Geometry: final body of the model. Coordinates: model frame, mm. Coordinates: 2 decimals unless noted, no trailing zeros. Write each loop counter-clockwise with the first axis right and the second up, starting at its lowest first coordinate (ties: lowest second). Pieces come first, ordered by that corner, then holes. Notation, with made-up numbers: (86.5, 27) - (132.5, 27) arc R30 ccw to (132.5, 54) - close; hole circle Ø8 at (-27, 10). An arc over 180 degrees is marked (long way). Answer as a JSON object with one key per item and string values. Group by question number.
Item 1: Section C-C on x = -45. Return loops of the section in (y, z), and give its area (3 significant figures).
Item 2: First-contact query: pin 1 Ø1 at (y, z) = (2, 96.5) entering from +X; pin 2 Ø1 at (y, z) = (0.5, 28) entering from -X. Flat tips, straight axial feed; report the tip coordinate or a pass-through.
Item 3: Line query: line 1 along Z through (x, y) = (-32.5, 0.6); line 2 along Z through (x, y) = (38, 0.8); line 3 along Z through (x, y) = (50.5, 1.35). Output: solid intervals per line, ascending. Write a range as from..to.
Item 4: Section D-D on y = 1.3. State how many separate pieces and enclosed holes the cut face has, and give its area (3 significant figures).
Item 5: Section B-B on z = 49.5. Return loops of the section in (x, y).
Item 6: Section A-A on x = -20. Return loops of the section in (y, z).
Autodesk Inventor part; units mm, degrees
ref_plane "YZ Plane" through (0, 0, 0) normal (1, 0, 0) x (0, 1, 0)
ref_plane "XZ Plane" through (0, 0, 0) normal (0, 1, 0) x (-1, 0, 0)
ref_plane "XY Plane" through (0, 0, 0) normal (0, 0, 1) x (1, 0, 0)
sketch "スケッチ1" plane through (0, 0, 0) normal (0, 1, 0) x (-1, 0, 0)
  circle A0 centre (0, 0) radius 130
  dimension "d0" = 260
extrude "プレート1" add sketch "スケッチ1" along normal blind 2
sketch "スケッチ4" plane through (0, 2, 0) normal (0, 1, 0) x (1, 0, 0)
  circle A0 centre (0, 0) radius 130
  line L0 (-106.1838, 75) -> (-60, 40)
  line L1 (-60, 40) -> (-60, -40)
  line L2 (-60, -40) -> (-106.1838, -75)
  point P0 (-60, 0)
  dimension "d17" = 40
  dimension "d18" = 75
  dimension "d19" = 60
extrude "押し出し2" cut sketch "スケッチ4" against normal through all contours L0 L1 L2 A0 picked at (-83.3333, 0)
sketch "スケッチ7" plane through (0, 2, 0) normal (0, 1, 0) x (1, 0, 0)
  arc A0 (-106.1838, -75) -> (-106.1838, 75) centre (0, 0) ccw
  line L0 (-48.7827, 120.5) -> (48.7827, 120.5)
  line L1 (-48.7827, -120.5) -> (48.7827, -120.5)
  line L2 (105, -76.6485) -> (105, 76.6485)
  dimension "d68" = 120.5
  dimension "d69" = 120.5
  dimension "d70" = 105
extrude "押し出し4" cut sketch "スケッチ7" against normal through all
fillet "フィレット4" radius 50 6 edges at (-48.7827, 1, 120.5) (48.7827, 1, 120.5) (105, 1, -76.6485) (105, 1, 76.6485) (-48.7827, 1, -120.5) (48.7827, 1, -120.5)
sketch "スケッチ9" plane through (0, 2, 0) normal (0, 1, 0) x (1, 0, 0)
  line L0 (101.5, -60) -> (101.5, 60) construction
  line L1 (101.5, -60) -> (221.5, -60) construction
  line L2 (105, -58.0948) -> (105, 58.0948) construction
  point P0 (0, 0)
  point P1 (101.5, 0)
  dimension "d71" = 120
  dimension "d72" = 90
  dimension "d73" = 3.5
hole "穴4" at (101.5, 2, 60) at (101.5, 2, -60) direction (0, -1, 0) diameter 3.5 depth 2 tip angle 118
sketch "スケッチ10" plane through (0, 2, 0) normal (0, 1, 0) x (1, 0, 0)
  line L0 (10, -105.5) -> (-10, -105.5) construction
  line L1 (-10, -105.5) -> (-10, 105.5) construction
  line L2 (-10, 105.5) -> (10, 105.5) construction
  line L3 (10, 105.5) -> (10, -105.5) construction
  line L4 (10, -105.5) -> (-10, 105.5) construction
  line L5 (-10, -105.5) -> (10, 105.5) construction
  point P0 (0, 0)
  dimension "d81" = 20
  dimension "d82" = 211
hole "穴5" at (-10, 2, 105.5) at (10, 2, 105.5) at (10, 2, -105.5) at (-10, 2, -105.5) direction (0, -1, 0) diameter 3.5 depth 2 tip angle 118
sketch "スケッチ11" plane through (0, 2, 0) normal (0, 1, 0) x (1, 0, 0)
  line L0 (-32.5, 116.5) -> (32.5, 116.5) construction
  line L1 (-32.5, 116.5) -> (32.5, 116.5) construction
  line L2 (37.812, 120.5) -> (-37.812, 120.5) construction
  point P0 (0, 0)
  point P1 (0, 116.5)
  dimension "d90" = 65
  dimension "d91" = 0
  dimension "d92" = 4
hole "穴6" at (32.5, 2, -116.5) at (-32.5, 2, -116.5) direction (0, -1, 0) diameter 3.5 end through all
mirror "ミラー3" about plane through (0, 0, 0) normal (0, 0, 1) of "穴6"
sketch "スケッチ12" plane through (0, 2, 0) normal (0, 1, 0) x (1, 0, 0)
  line L0 (-50, 10) -> (-50, -10) construction
  line L1 (-50, 10) -> (-30, 10) construction
  line L2 (-60, 40) -> (-60, -40) construction
  point P0 (0, 0)
  point P1 (-50, 0)
  dimension "d100" = 20
  dimension "d101" = 90
  dimension "d102" = 10
hole "穴7" at (-50, 2, 10) at (-50, 2, -10) direction (0, -1, 0) diameter 3.5 end through all
sketch "スケッチ13" plane through (0, 2, 0) normal (0, 1, 0) x (1, 0, 0)
  line L0 (-10, 40) -> (40, 40) construction
  line L1 (-10, 10) -> (40, 10)
  line L2 (40, 70) -> (-10, 70)
  arc A0 (-10, 70) -> (-10, 10) centre (-10, 40) ccw
  arc A1 (40, 10) -> (40, 70) centre (40, 40) ccw
  point P0 (0, 0)
  point P1 (15, 40)
  dimension "d110" = 40
  dimension "d111" = 60
  dimension "d112" = 50
  dimension "d113" = 15
extrude "押し出し5" cut sketch "スケッチ13" against normal through all
sketch "スケッチ14" plane through (0, 2, 0) normal (0, 1, 0) x (1, 0, 0)
  line L0 (72.6777, 95.6777) -> (55, 78) construction
  line L1 (75.5061, 92.8492) -> (57.8284, 75.1716)
  line L2 (52.1716, 80.8284) -> (69.8492, 98.5061)
  arc A0 (75.5061, 92.8492) -> (69.8492, 98.5061) centre (72.6777, 95.6777) ccw
  arc A1 (52.1716, 80.8284) -> (57.8284, 75.1716) centre (55, 78) ccw
  line L3 (-10, 70) -> (40, 70)
  point P0 (0, 0)
  point P1 (63.8388, 86.8388)
  dimension "d116" = 135
  dimension "d117" = 8
  dimension "d118" = 25
  dimension "d119" = 4
  dimension "d120" = 15
extrude "押し出し6" cut sketch "スケッチ14" against normal through all
pattern_linear "矩形状パターン1" count 6 spacing 25 along (-1, 0, 0) of "押し出し6"
mirror "ミラー4" about plane through (0, 0, 0) normal (0, 0, 1) of "押し出し5", "押し出し6", "矩形状パターン1"
sketch "スケッチ15" plane through (0, 0, 0) normal (0, -1, 0) x (1, 0, 0)
  arc A0 (73.6766, 79.5874) -> (73.6766, 77.4126) centre (74.2931, 78.5) ccw
  arc A1 (74.9095, -79.5874) -> (74.9095, -77.4126) centre (74.2931, -78.5) ccw
  point P0 (0, 0)
hole "穴8" at (74.2931, 0, -78.5) at (74.2931, 0, 78.5) direction (0, 1, 0) diameter 3.5 end through all
sketch "スケッチ16" plane through (0, 2, 0) normal (0, 1, 0) x (1, 0, 0)
  arc A0 (-61.4446, 114.5625) -> (-106.1838, 75) centre (0, 0) ccw
  arc A1 (-106.1838, -75) -> (-61.4446, -114.5625) centre (0, 0) ccw
  line L0 (-102.4695, 80) -> (-102.4695, -80)
  line L1 (-102.4695, 80) -> (57.5305, 80) construction
  line L2 (-106.1838, 75) -> (-60, 40)
  line L3 (-60, -40) -> (-106.1838, -75)
  point P0 (-102.4695, 72.1852)
  point P1 (-102.4695, -72.1852)
  dimension "d133" = 160
  dimension "d134" = 90
extrude "押し出し7" cut sketch "スケッチ16" against normal through all
sketch "スケッチ17" plane through (0, 2, 0) normal (0, 1, 0) x (1, 0, 0)
  line L0 (-92.9695, 76.5) -> (-82.9695, 76.5) construction
  line L1 (-82.9695, 76.5) -> (-82.9695, -76.5) construction
  line L2 (-82.9695, -76.5) -> (-92.9695, -76.5) construction
  line L3 (-92.9695, -76.5) -> (-92.9695, 76.5) construction
  line L4 (-92.9695, 76.5) -> (-82.9695, -76.5) construction
  line L5 (-82.9695, 76.5) -> (-92.9695, -76.5) construction
  line L6 (-102.4695, 80) -> (-102.4695, 72.1852) construction
  point P0 (0, 0)
  point P1 (-87.9695, 0)
  dimension "d137" = 10
  dimension "d138" = 153
  dimension "d139" = 9.5
hole "穴9" at (-92.9695, 2, -76.5) at (-82.9695, 2, -76.5) at (-92.9695, 2, 76.5) at (-82.9695, 2, 76.5) direction (0, -1, 0) diameter 3.5 end through all
fillet "フィレット5" radius 2 6 edges at (-102.4695, 1, -72.1852) (-102.4695, 1, 80) (-102.4695, 1, -80) (-60, 1, -40) (-60, 1, 40) (-102.4695, 1, 72.1852)
sketch "スケッチ18" plane through (0, 2, 0) normal (0, 1, 0) x (1, 0, 0)
  line L0 (105, -58.0948) -> (105, 58.0948)
  line L1 (-60, 39.0062) -> (-60, -39.0062)
  line L2 (-60, 0) -> (105, 0) construction
  circle A0 centre (-50, 10) radius 1.75 construction
  line L3 (95, -10) -> (-50, -10) construction
  line L4 (-50, -10) -> (-50, 10) construction
  line L5 (-50, 10) -> (95, 10) construction
  line L6 (95, 10) -> (95, -10) construction
  line L7 (95, -10) -> (-50, 10) construction
  line L8 (-50, -10) -> (95, 10) construction
  line L9 (52.5, -5) -> (-7.5, -5) construction
  line L10 (-7.5, -5) -> (-7.5, 5) construction
  line L11 (-7.5, 5) -> (52.5, 5) construction
  line L12 (52.5, 5) -> (52.5, -5) construction
  line L13 (52.5, -5) -> (-7.5, 5) construction
  line L14 (-7.5, -5) -> (52.5, 5) construction
  point P0 (0, 0)
  point P1 (22.5, 0)
  point P2 (22.5, 0)
  dimension "d148" = 60
  dimension "d149" = 10
hole "穴10" at (95, 2, 10) at (95, 2, -10) at (52.5, 2, 5) at (52.5, 2, -5) at (-7.5, 2, -5) at (-7.5, 2, 5) direction (0, -1, 0) diameter 3.5 end through all
sketch "スケッチ19" plane through (0, 2, 0) normal (0, 1, 0) x (1, 0, 0)
  line L0 (-60, 39.0062) -> (-60, -39.0062)
  arc A0 (-60, 39.0062) -> (-60.792, 40.6002) centre (-62, 39.0062) ccw
  line L1 (-101.6775, 71.5849) -> (-60.792, 40.6002)
  arc A1 (-102.4695, 73.1789) -> (-101.6775, 71.5849) centre (-100.4695, 73.1789) ccw
  line L2 (-102.4695, 79.3088) -> (-102.4695, 73.1789)
  arc A2 (-102.0393, 80.548) -> (-102.4695, 79.3088) centre (-100.4695, 79.3088) ccw
  arc A3 (-61.4446, 114.5625) -> (-102.0393, 80.548) centre (0, 0) ccw
  arc A4 (-37.812, 120.5) -> (-61.4446, 114.5625) centre (-37.812, 70.5) ccw
  line L3 (37.812, 120.5) -> (-37.812, 120.5)
  arc A5 (61.4446, 114.5625) -> (37.812, 120.5) centre (37.812, 70.5) ccw
  arc A6 (89.375, 94.404) -> (61.4446, 114.5625) centre (0, 0) ccw
  arc A7 (105, 58.0948) -> (89.375, 94.404) centre (55, 58.0948) ccw
  line L4 (105, -58.0948) -> (105, 58.0948)
  line L5 (-60, 0) -> (105, 0)
extrude "押し出し8" cut sketch "スケッチ19" against normal through all
fillet "フィレット6" radius 1 2 edges at (-60, 1, 0) (105, 1, 0)
sketch "スケッチ20" plane through (0, 0, 0) normal (0, 1, 0) x (-1, 0, 0)
  line L0 (115.5948, 100.5744) -> (-72.3437, 168.9784)
  line L1 (-72.3437, 168.9784) -> (-130.4866, 9.2322)
  line L2 (-130.4866, 9.2322) -> (57.4519, -59.1718)
  line L3 (57.4519, -59.1718) -> (115.5948, 100.5744)
  line L4 (-104, 0) -> (59, 0)
  point P0 (0, 0)
  dimension "d161" = 200
  dimension "d162" = 20
equation "\"d79\" = Thickness"
equation "\"d88\" = Thickness"
equation "\"d98\" = Thickness"
equation "\"d108\" = Thickness"
equation "\"d131\" = Thickness"
equation "\"d145\" = Thickness"
equation "\"d155\" = Thickness"
equation "\"d1\" = Thickness"
equation "\"BendRadius\" = Thickness"
equation "\"BendReliefWidth\" = Thickness"
equation "\"BendReliefDepth\" = 0.5 * Thickness"
equation "\"CornerReliefSize\" = 4 * Thickness"
equation "\"MinimumRemnant\" = 2 * Thickness"
equation "\"TransitionRadius\" = BendRadius"
equation "\"JacobiRadiusSize\" = BendRadius"
equation "\"GapSize\" = Thickness"
properties part number "T2.0_frame-base3"
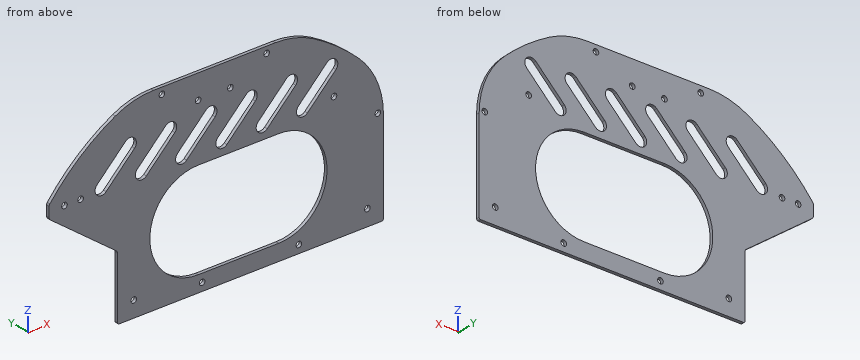
Checks:
{
 "1": {"outline": "(0, 0) - (2, 0) - (2, 74) - (0, 74) - close; (0, 83.66) - (2, 83.66) - (2, 119.98) - (0, 119.98) - close", "area": "221 mm^2"},
 "2": {"pin 1": "x = 87.66", "pin 2": "x = -60"},
 "3": {"line 1": "0..20.16, 59.84..84.84, 96.16..114.75, 118.25..120.5", "line 2": "0..10, 70..80.34, 91.66..120.5", "line 3": "0..11.9, 68.1..92.84, 98.51..118.86"},
 "4": {"separate pieces": "1", "enclosed holes": "19", "area": "13,200 mm^2"},
 "5": {"outline": "(-72.54, 0) - (-38.46, 0) - (-38.46, 2) - (-72.54, 2) - close; (68.46, 0) - (105, 0) - (105, 2) - (68.46, 2) - close"},
 "6": {"outline": "(0, 0) - (2, 0) - (2, 11.72) - (0, 11.72) - close; (0, 68.28) - (2, 68.28) - (2, 74) - (0, 74) - close; (0, 83.66) - (2, 83.66) - (2, 120.5) - (0, 120.5) - close"}
}
